```python
from build123d import *

# Parameters (mm, degrees)
SKETCH008_W             = 14
SKETCH008_H             = 14
SKETCH008_R             = 3.8
PAD007_DEPTH            = 6
PAD008_DEPTH            = 14
PAD009_DEPTH            = 3
PAD010_DEPTH            = 3
BODY002_PLACEMENT_ANGLE = 315


with BuildPart() as part:
    # Sketch008 → Pad007 (new body)
    with BuildSketch(Plane.YZ):
        with Locations((-12, 7)):
            Rectangle(SKETCH008_W, SKETCH008_H)
        with Locations((-12, 7)):
            Circle(SKETCH008_R, mode=Mode.SUBTRACT)
    extrude(amount=PAD007_DEPTH)

    # Sketch009 → Pad008 (join)
    with BuildSketch(Plane.XZ.offset(5)):
        Polygon((0, 0), (21.213203, 0), (8.485281, -12.727922), align=None)
    extrude(amount=PAD008_DEPTH)

    # Sketch010 → Pad009 (join)
    with BuildSketch(Plane.XZ.offset(5)):
        Polygon((0, 14), (7.213203, 14), (21.213203, 0), (8.485281, -12.727922), (-5.6, 8.4), align=None)
    extrude(amount=-PAD009_DEPTH)

    # Sketch011 → Pad010 (join)
    with BuildSketch(Plane.XZ.offset(19)):
        Polygon((0, 14), (7.213203, 14), (21.213203, 0), (8.485281, -12.727922), (-5.6, 8.4), align=None)
    extrude(amount=PAD010_DEPTH)


with BuildPart() as part_1:
    # Body002 placement: moved
    add(part.part.moved(Location((-17, 22, -15))).rotate(Axis((-17, 22, -15), (0, 1, 0)), BODY002_PLACEMENT_ANGLE))


solid = part_1.part
```
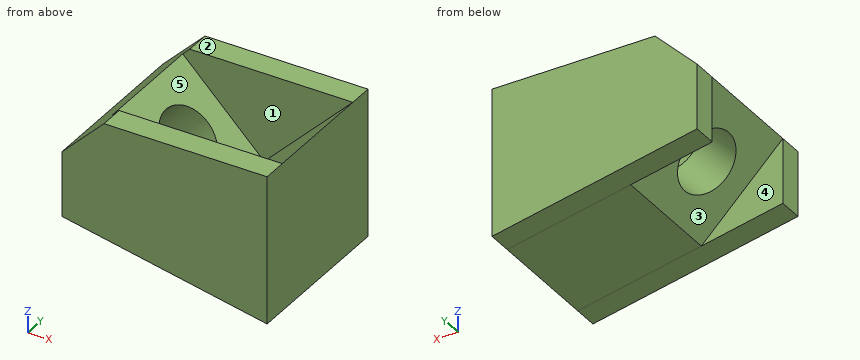
Source: CAD feature listing. Evaluate the final solid. Frame: model axes, mm. Face numbers are marked on the shaded views. A direction names the side the tool comes from. Give positions to 0.01 mm unless a question says otherwise; leave off trailing zeros. Order: outer loops, then holes, each group sorted by start corner. A loop starts at its lowest first (then second) coordinate and runs counter-clockwise, first axis right, second up.
(1) Section query D-D (y = 14.75). Return the cut outline in (x, z), plus the area to 3 significant figures.
(2) Section query C-C (z = -2). Return the cut outline in (x, y), plus the area to 3 significant figures.
(3) Pull-direction query (X, two-part tool) for the marked faces 3, 4 and 5; classes: +X half, -X half, draft (parallel to the pull), parting line (faces both ways), or undercut.
(4) Section query A-A (x = -5). Return the cut outline in (y, z).
(5) Material intervals for line 1 along Y through (x, z) = (-25.25, -12); line 2 along X through (y, z) = (7, -14); line 3 along X through (y, z) = (3.5, -10.5), sorted ascending.
(6) Access query for the marked faces 1 and 2. Directions: +Z, -Z, +X, -X, +Y, -Y. A direction counts if a zero-diameter tool reaches every point of the face in a straight line with its end or side. Return the directions, or none.
(7) Contact query for flat-ended pins moving along their axis: P1, Ø1.5, axis at x = -8.5, z = -5, coming from the -Y side; P2, Ø3, axis at x = -18.5, y = 14, coming from the +Z side. Output: stop coordinate, or through.
(8) Section query B-B (y = 7.25). Return the cut outline in (x, z), plus the area to 3 significant figures.
Outcome:
1. outline: (-26.9, -5.1) - (-17, -15) - (-2, -18) - (-2, 0) - (-12.76, -10.76) - (-22.66, -0.86) - close
1. area: 219 mm2
2. outline: (-23.8, 0) - (-2, 0) - (-2, 20) - (-23.8, 20) - close; hole (-21.51, 3) - (-4, 3) - (-4, 17) - (-21.51, 17) - close
2. area: 191 mm2
3. face 3: -X half
3. face 4: draft
3. face 5: undercut
4. outline: (0, -17.4) - (20, -17.4) - (20, 0) - (17, 0) - (17, -3) - (3, -3) - (3, 0) - (0, 0) - close
5. line 1: y = 0 to 3, 17 to 20
5. line 2: x = -18 to -2
5. line 3: x = -21.5 to -13.01, -12.5 to -2
6. face 1: +Z
6. face 2: +Z, +X, -X, +Y, -Y
7. P1: stops at y = 0
7. P2: stops at z = -3.51
8. outline: (-26.9, -5.1) - (-23.8, -8.2) - (-19.56, -3.95) - (-22.66, -0.86) - close; (-20.1, -11.9) - (-17, -15) - (-2, -18) - (-2, 0) - (-12.76, -10.76) - (-15.85, -7.66) - close
8. area: 188 mm2
